Autodesk Inventor part; units mm, degrees
ref_plane "YZ Plane" through (0, 0, 0) normal (1, 0, 0) x (0, 1, 0)
ref_plane "XZ Plane" through (0, 0, 0) normal (0, 1, 0) x (-1, 0, 0)
ref_plane "XY Plane" through (0, 0, 0) normal (0, 0, 1) x (1, 0, 0)
sketch "Sketch2" plane through (0, 0, 0) normal (0, 0, 1) x (1, 0, 0)
  line L0 (0, 0) -> (0, 4)
  line L1 (0, 4) -> (1.5, 4)
  line L2 (0, 0) -> (5.5, 0)
  line L3 (5.5, 0) -> (5.5, 6)
  line L4 (1.5, 4) -> (1.5, 1)
  line L5 (1.5, 1) -> (3.75, 1)
  line L6 (3.75, 1) -> (3.75, 6)
  line L7 (3.75, 6) -> (-1.8459, 7.5)
  line L8 (-1.8459, 7.5) -> (3.75, 9)
  line L9 (5.5, 6) -> (-0.0959, 7.5)
  line L10 (-0.0959, 7.5) -> (5.5, 9)
  line L11 (5.5, 9) -> (0.1177, 10.5)
  line L12 (3.75, 9) -> (-1.6323, 10.5)
  line L13 (-1.6323, 10.5) -> (3.75, 12)
  line L14 (0.1177, 10.5) -> (5.5, 12)
  line L15 (5.5, 12) -> (0.1177, 13.5)
  line L16 (3.75, 12) -> (-1.6323, 13.5)
  line L17 (-1.6323, 13.5) -> (3.75, 15)
  line L18 (0.1177, 13.5) -> (5.5, 15)
  line L19 (5.5, 15) -> (0.1177, 16.5)
  line L20 (3.75, 15) -> (-1.6323, 16.5)
  line L21 (-1.6323, 16.5) -> (3.75, 18)
  line L22 (0.1177, 16.5) -> (5.5, 18)
  line L23 (5.5, 18) -> (0.1177, 19.5)
  line L24 (3.75, 18) -> (-1.6323, 19.5)
  line L25 (-1.6323, 19.5) -> (3.75, 21)
  line L26 (0.1177, 19.5) -> (5.5, 21)
  line L27 (5.5, 21) -> (0.1177, 22.5)
  line L28 (3.75, 21) -> (-1.6323, 22.5)
  line L29 (-1.6323, 22.5) -> (3.75, 24)
  line L30 (0.1177, 22.5) -> (5.5, 24)
  line L31 (6.6857, 15) -> (8.563, 15) construction
  line L32 (0, 30) -> (0, 26)
  line L33 (0, 26) -> (1.5, 26)
  line L34 (0, 30) -> (5.5, 30)
  line L35 (5.5, 30) -> (5.5, 24)
  line L36 (1.5, 26) -> (1.5, 29)
  line L37 (1.5, 29) -> (3.75, 29)
  line L38 (3.75, 29) -> (3.75, 24)
  dimension "d14" = 4
  dimension "d15" = 1.5
  dimension "d16" = 5.5
  dimension "d17" = 6
  dimension "d18" = 3
  dimension "d19" = 2.25
  dimension "d24" = 5
  dimension "d25" = 3
  dimension "d28" = 1.5
  dimension "d29" = 0
  dimension "d37" = 15.573
  dimension "d38" = 15
  dimension "d39" = 3.063
  dimension "d40" = 1.1857
extrude "Extrusion2" add sketch "Sketch2" along normal blind 5
equation "\"d28\" = 0.5 * d25"
properties part number "Spring Mk 1.1"
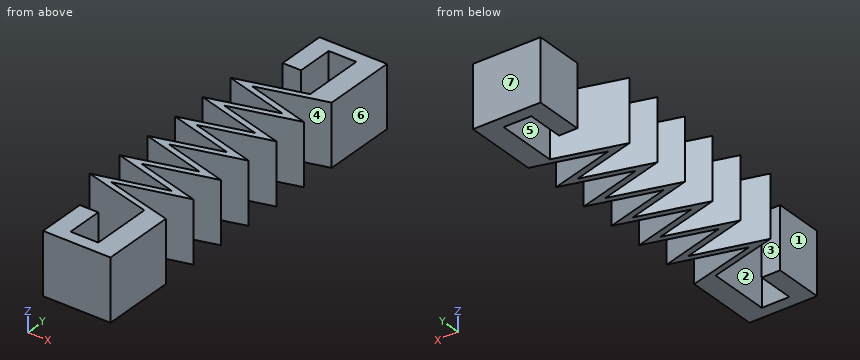
Model file for the job. Use its own axes, mm. Face numbers are marked on the shaded views. A direction names the side the tool comes from. Give positions to 0.01 mm unless a question says otherwise; leave off trailing zeros. Order: outer loops, then holes, each group sorted by start corner. A loop starts at its lowest first (then second) coordinate and runs counter-clockwise, first axis right, second up. Notation, with made-up numbers: (-27.5, 42.5) - (-2.5, 42.5) arc R24 ccw to (-2.5, 79.5) - close; hole circle Ø2 at (32.25, 70). An arc over 180 degrees is marked (long way). Write item = value, one per line. Start each with the question number.
1. Cut at C-C, the plane x = 4.75. List the corners of the cut face in (y, z), and give its area (3 significant figures).
2. Which spindle directions (+Z, -Z, +X, -X, +Y, -Y) get a long thin tool onto all of the face, cutting with end or side? Do the marked faces 1, 2, 3 and 4. Say none if no direction does.
3. Cut at D-D, the plane y = 12.75. List the corners of the cut face in (x, z), and give its area (3 significant figures).
4. Probe line 1 along X through (y, z) = (28, 1.95); line 2 along X through (y, z) = (5, 1.5). List the from-to ranges inside material, lowest first.
5. Cut at A-A, the plane y = 2.5. List the corners of the cut face in (x, z).
6. Cut at B-B, the plane x = -1. List the corners of the cut face in (y, z), and give its area (3 significant figures).
7. Two-plate mould, pull along Y, no slides. Class the marked faces 5, 6 and 7: pulls with the +Y half, pulls with the -Y half, needs draft (parallel to the pull), parting line crosses it, or undercut.
Taken from the geometry:
q1.outline = (0, 0) - (6.2, 0) - (6.2, 5) - (0, 5) - close; (8.8, 0) - (9.21, 0) - (9.21, 5) - (8.8, 5) - close; (11.79, 0) - (12.21, 0) - (12.21, 5) - (11.79, 5) - close; (14.79, 0) - (15.21, 0) - (15.21, 5) - (14.79, 5) - close; (17.79, 0) - (18.21, 0) - (18.21, 5) - (17.79, 5) - close; (20.79, 0) - (21.21, 0) - (21.21, 5) - (20.79, 5) - close; (23.79, 0) - (30, 0) - (30, 5) - (23.79, 5) - close
q1.area = 72.5 mm²
q2.face_1 = +Z, -Z, -X, -Y
q2.face_2 = +Z, -Z
q2.face_3 = +Z, -Z, -X
q2.face_4 = +Z, -Z, +X
q3.outline = (1.06, 0) - (2.81, 0) - (2.81, 5) - (1.06, 5) - close
q3.area = 8.75 mm²
q4.line_1 = 0 to 1.5, 3.75 to 5.5
q4.line_2 = 3.75 to 5.5
q5.outline = (0, 0) - (1.5, 0) - (1.5, 5) - (0, 5) - close; (3.75, 0) - (5.5, 0) - (5.5, 5) - (3.75, 5) - close
q6.outline = (7.27, 0) - (7.73, 0) - (7.73, 5) - (7.27, 5) - close; (10.32, 0) - (10.68, 0) - (10.68, 5) - (10.32, 5) - close; (13.32, 0) - (13.68, 0) - (13.68, 5) - (13.32, 5) - close; (16.32, 0) - (16.68, 0) - (16.68, 5) - (16.32, 5) - close; (19.32, 0) - (19.68, 0) - (19.68, 5) - (19.32, 5) - close; (22.32, 0) - (22.68, 0) - (22.68, 5) - (22.32, 5) - close
q6.area = 11.1 mm²
q7.face_5 = undercut
q7.face_6 = needs draft
q7.face_7 = pulls with the +Y half
